from build123d import *

# Parameters (mm, degrees)
CORTAR_EXTRUIR3_DEPTH   = 31.75
SALIENTE_EXTRUIR1_DEPTH = 48.26
SALIENTE_EXTRUIR2_START = -29.633333
CROQUIS7_W              = 171.45
CROQUIS7_H              = 177.8
SALIENTE_EXTRUIR2_DEPTH = 29.633333
CORTAR_EXTRUIR4_REACH   = 466.994
CROQUIS8_W              = 100.33
CROQUIS8_H              = 78.74


with BuildPart() as part:
    # Croquis2 → Recubrir1 section 0
    with BuildSketch(Plane(origin=(0, 0, 0), x_dir=(1, 0, 0), z_dir=(0, 1, 0))):
        with BuildLine():
            Line((212.725, -139.7), (-212.725, -139.7))
            Line((-212.725, -139.7), (-212.725, 139.7))
            Line((-212.725, 139.7), (212.725, 139.7))
            Line((212.725, 139.7), (212.725, -139.7))
        make_face()
    # Croquis3 → Recubrir1 section 1
    with BuildSketch(Plane(origin=(0, 304.8, 0), x_dir=(1, 0, 0), z_dir=(0, 1, 0))):
        with BuildLine():
            Line((111.125, -88.9), (-111.125, -88.9))
            Line((-111.125, -88.9), (-111.125, 88.9))
            Line((-111.125, 88.9), (111.125, 88.9))
            Line((111.125, 88.9), (111.125, -88.9))
        make_face()
    loft()

    # Croquis5 → Cortar-Extruir3 (cut)
    with BuildSketch(Plane(origin=(0, 304.8, 0), x_dir=(1, 0, 0), z_dir=(0, 1, 0))):
        Polygon((171.921254814, -45.72), (34.925, -45.72), (34.925, -107.229562049), (-34.925, -107.229562049), (-34.925, -45.72), (-171.921254814, -45.72), (-171.921254814, 45.72), (-34.925, 45.72), (-34.925, 107.229562049), (34.925, 107.229562049), (34.925, 45.72), (171.921254814, 45.72), align=None)
    extrude(amount=-CORTAR_EXTRUIR3_DEPTH, mode=Mode.SUBTRACT)

    # Croquis6 → Saliente-Extruir1 (add)
    with BuildSketch(Plane(origin=(-212.725, 0, 0), x_dir=(0, 0, -1), z_dir=(1, 0, 0))):
        Polygon((139.7, 0), (0, 144.78), (-139.7, 0), align=None)
    extrude(amount=SALIENTE_EXTRUIR1_DEPTH)

    # Croquis7 → Saliente-Extruir2 (add)
    with BuildSketch(Plane.XY.offset(139.7).offset(SALIENTE_EXTRUIR2_START)):
        with Locations((0, 88.9)):
            Rectangle(CROQUIS7_W, CROQUIS7_H)
    extrude(amount=SALIENTE_EXTRUIR2_DEPTH)

    # Cortar-Extruir4: up to this plane
    cortar_extruir4_end = Plane(origin=(0, 22.654054054, -135.924324324), z_dir=(0, -0.16439898730535737, 0.9863939238321437))
    # Croquis8 → Cortar-Extruir4 (cut, up to the surface)
    with BuildSketch(Plane.XY.offset(139.7), mode=Mode.PRIVATE) as cortar_extruir4_sk1:
        with Locations((0, 39.37)):
            Rectangle(CROQUIS8_W, CROQUIS8_H)
    cortar_extruir4_tool1 = split(extrude(cortar_extruir4_sk1.sketch, amount=-CORTAR_EXTRUIR4_REACH, mode=Mode.PRIVATE), bisect_by=cortar_extruir4_end, keep=Keep.BOTH, mode=Mode.PRIVATE)
    add(cortar_extruir4_tool1.solids().sort_by_distance((0, 39.37, 139.7))[0], mode=Mode.SUBTRACT)


solid = part.part
Geometry check sheet. Reference: the model listing, model coordinates, mm. A direction names the side the tool comes from. Coordinates: 2 decimals unless noted, no trailing zeros. Use a Markdown table: item, result. Add a question column.
1. Mould release check, pull along Z, two halves, no side actions. Record for faces 5 (the face through (-199.657, 103.55, -39.783)), 6 (the face through (85.725, 127, 131)), 7 (the face through (79, 289, 45.72)): pulls with the +Z half, pulls with the -Z half, needs draft (parallel to the pull), parting line crosses it, or undercut.
2. Material ranges on L1, parallel to Y at x = -59, z = 2.5; L2, parallel to X at y = 45, z = 19 (3 decimals); L3, parallel to X at y = 26, z = 42 (3 decimals), recorded low to high.
3. Set-up check for faces 1 (the face through (-1, 177.8, 125)), 2 (the face through (-194.3, 89.49, 53.35)), 3 (the face through (34.925, 289, 70)), 4 (the face through (-50.165, 39, 2)): record each of +Z, -Z, +X, -X, +Y, -Y from which the full face is reachable in a straight line by a thin tool's end or side.
4. Go/stop test with flat-tipped pins: pin 1 Ø3 at (x, z) = (-22.5, -21.5) entering from +Y; pin 2 Ø1.5 at (x, y) = (-107, 190.5) entering from -Z; pin 3 Ø9 at (y, z) = (124.5, 119) entering from +X (3 decimals). Record where each tip stops, or that it passes through.
Filled sheet:
| question | item | result |
|---|---|---|
| 1 | face 5 | pulls with the -Z half |
| 1 | face 6 | needs draft |
| 1 | face 7 | undercut |
| 2 | L1 | 0 to 273.05 |
| 2 | L2 | -212.725 to -50.165, 50.165 to 197.725 |
| 2 | L3 | -212.725 to -50.165, 50.165 to 204.058 |
| 3 | face 1 | +Z, +X, -X, +Y |
| 3 | face 2 | +Z, -X, +Y |
| 3 | face 3 | +Z, -Z, +Y |
| 3 | face 4 | +Z, -Z, -Y |
| 4 | pin 1 | y = 273.05 |
| 4 | pin 2 | z = -108.08 |
| 4 | pin 3 | x = 172.725 |
